```python
from build123d import *

# Parameters (mm, degrees)
SKETCH_1_W          = 20
SKETCH_1_H          = 20
EXTRUDE_1_DEPTH     = 40
SKETCH_2_R          = 2.15
CUT_EXTRUDE_1_DEPTH = 40
FILLET_2_R          = 1


with BuildPart() as part:
    # 草图1 → 凸台-拉伸1 (new body)
    with BuildSketch(Plane.XY):
        with Locations((10, 10)):
            Rectangle(SKETCH_1_W, SKETCH_1_H)
    extrude(amount=EXTRUDE_1_DEPTH)

    # 草图2 → 切除-拉伸1 (cut)
    with BuildSketch(Plane(origin=(0, 20, 0), x_dir=(1, 0, 0), z_dir=(0, 1, 0))):
        with Locations(Location((10, -30, 0), (0, 0, 270))):
            Circle(SKETCH_2_R)
        with Locations(Location((10, -10, 0), (0, 0, 270))):
            Circle(SKETCH_2_R)
    extrude(amount=-CUT_EXTRUDE_1_DEPTH, mode=Mode.SUBTRACT)

    # 圆角2
    fillet_2_edges = [part.edges().sort_by_distance(p)[0] for p in [
        (20, 10, 40),
        (10, 20, 40),
        (0, 10, 40),
        (10, 20, 0),
        (20, 10, 0),
        (10, 0, 0),
        (0, 10, 0),
        (0, 20, 20),
        (20, 20, 20),
        (20, 0, 20),
        (0, 0, 20),
        (10, 0, 40),
    ]]
    fillet(fillet_2_edges, radius=FILLET_2_R)


solid = part.part
```
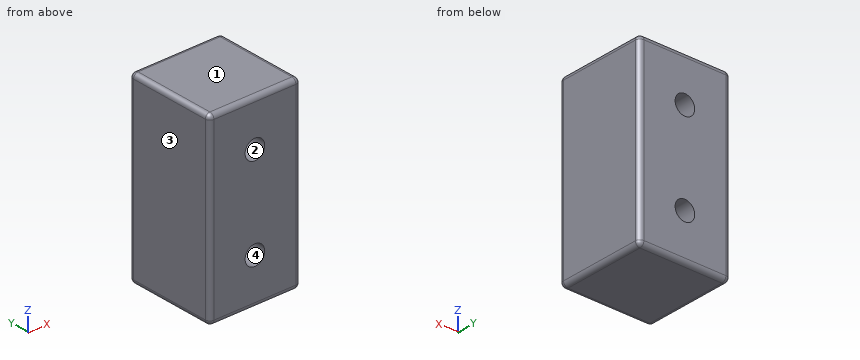
Model file for the job. Use its own axes, mm. Face numbers are marked on the shaded views. Give positions to 0.01 mm unless a question says otherwise; leave off trailing zeros. Order: outer loops, then holes, each group sorted by start corner. A loop starts at its lowest first (then second) coordinate and runs counter-clockwise, first axis right, second up.
1) Saw through at B-B, the plane y = 4. Write the cut outline in (x, z), then the cut area to 3 significant figures.
2) Wall check: probe 1 along Z at (x, y) = (11.75, 16.5); probe 2 along X at (y, z) = (7, 30); probe 3 along Z at (x, y) = (10.25, 1.5). Give the ranges that are in metal, low to high.
3) Saw through at A-A, the plane x = 10. Write the cut outline in (y, z), then the cut area to 3 significant figures.
4) Saw through at C-C, the plane z = 30. Write the cut outline in (x, y).
5) Mould opens along Z. For the marked faces 1, 2, 3 and 4 say: +Z half, -Z half, draft (parallel to the pull), parting line (faces both ways), or undercut.
6) Pin check, flat tip, straight feed: pin 1 (4 mm diameter, centred on x = 10, z = 30, fed in from -Y). Stop position of the tip, or through.
Computed:
1. outline: (0, 1) arc R1 ccw to (1, 0) - (19, 0) arc R1 ccw to (20, 1) - (20, 39) arc R1 ccw to (19, 40) - (1, 40) arc R1 ccw to (0, 39) - close; hole circle Ø4.3 at (10, 10); hole circle Ø4.3 at (10, 30)
1. area: 770 mm2
2. probe 1: z = 0 to 8.75, 11.25 to 28.75, 31.25 to 40
2. probe 2: x = 0 to 7.85, 12.15 to 20
2. probe 3: z = 0 to 7.86, 12.14 to 27.86, 32.14 to 40
3. outline: (0, 1) arc R1 ccw to (1, 0) - (19, 0) arc R1 ccw to (20, 1) - (20, 7.85) - (0, 7.85) - close; (0, 12.15) - (20, 12.15) - (20, 27.85) - (0, 27.85) - close; (0, 32.15) - (20, 32.15) - (20, 39) arc R1 ccw to (19, 40) - (1, 40) arc R1 ccw to (0, 39) - close
3. area: 627 mm2
4. outline: (0, 1) arc R1 ccw to (1, 0) - (7.85, 0) - (7.85, 20) - (1, 20) arc R1 ccw to (0, 19) - close; (12.15, 0) - (19, 0) arc R1 ccw to (20, 1) - (20, 19) arc R1 ccw to (19, 20) - (12.15, 20) - close
5. face 1: +Z half
5. face 2: undercut
5. face 3: draft
5. face 4: undercut
6. pin 1: passes through
